Part print with two shaded views. Sizes in mm from the minimum x, y, z corner. A direction names the side the tool comes from. Round coordinates to 2 decimals unless told otherwise and drop trailing zeros. Write each loop counter-clockwise with the first axis right and the second up, starting at its lowest first coordinate (ties: lowest second). Pieces come first, ordered by that corner, then holes. Notation, with made-up numbers: (54.25, 77) -> (86.25, 77) arc R15 ccw to (86.25, 96) -> close; hole circle Ø5 at (70.5, -25). An arc over 180 degrees is marked (long way). Answer in a Markdown table with one row per item.
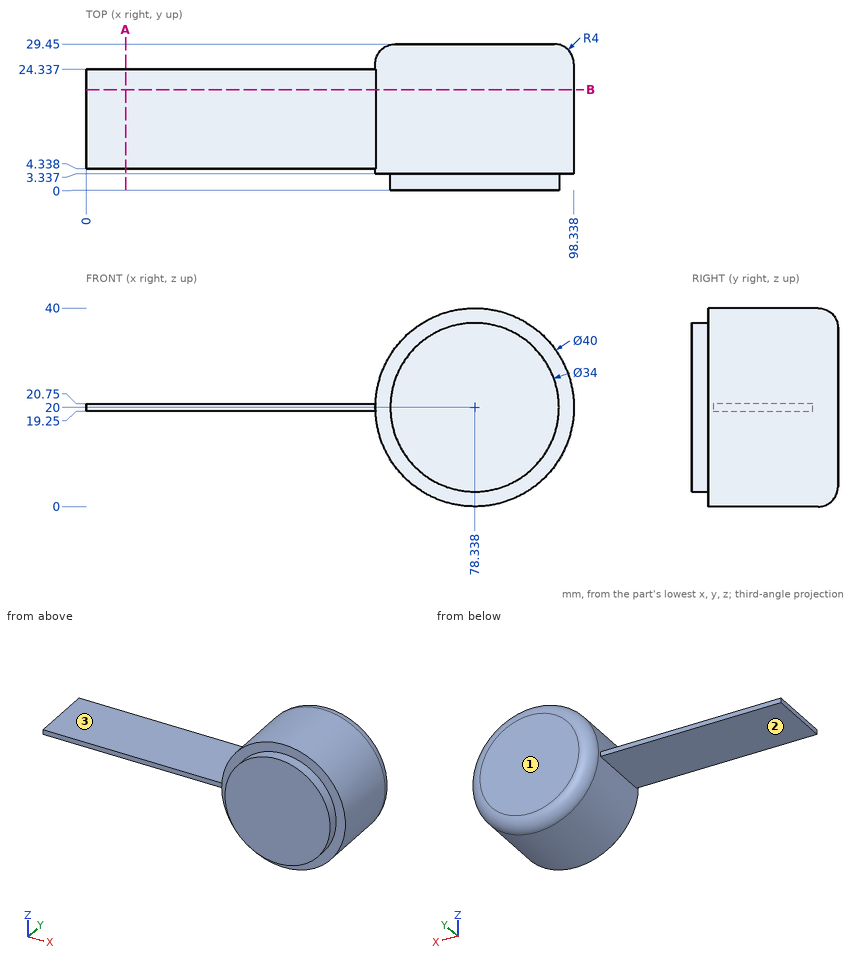
Q1. Wall check: line 1 (Z direction, x = 17, y = 14); line 2 (Z direction, x = 78, y = 23); line 3 (Y direction, x = 52, z = 19.5). Give the ranges that are in metal, low to high. Write a range as [from, to].
A:
| item | result |
|---|---|
| line 1 | [19.25, 20.75] |
| line 2 | [0, 40] |
| line 3 | [4.34, 24.34] |
Q2. Saw through at A-A on x = 8. Write the cut outline in (y, z).
A:
| item | result |
|---|---|
| outline | (4.34, 19.25) -> (24.34, 19.25) -> (24.34, 20.75) -> (4.34, 20.75) -> close |
Q3. Which spindle directions (+Z, -Z, +X, -X, +Y, -Y) get a long thin tool onto all of the face, cutting with end or side? Do the marked faces 1, 2 and 3. Say none if no direction does.
A:
| item | result |
|---|---|
| face 1 | +Z, -Z, +X, -X, +Y |
| face 2 | -Z, -X, +Y, -Y |
| face 3 | +Z, -X, +Y, -Y |
Q4. Drop flat-ended pins along their axis: P1, Ø10, axis at x = 78, y = 17.5, coming from the +Z side; P2, Ø6, axis at x = 17, y = 9.5, coming from the -Z side; P3, Ø1.5, axis at x = 23.5, y = 15, coming from the +Z side. Give the stop position or say it passes through.
A:
| item | result |
|---|---|
| P1 | z = 40 |
| P2 | z = 19.25 |
| P3 | z = 20.75 |
Q5. Saw through at B-B on y = 20.25. Write the cut outline in (x, z).
A:
| item | result |
|---|---|
| outline | (0, 19.25) -> (58.35, 19.25) arc R20 ccw (long way) to (58.35, 20.75) -> (0, 20.75) -> close |
